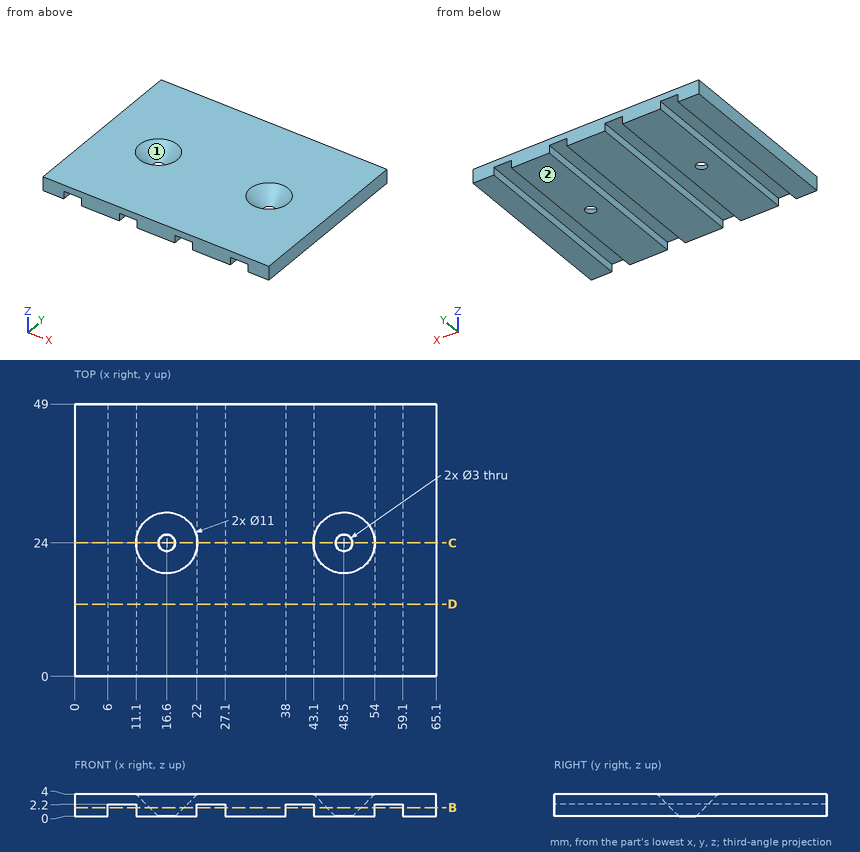
Study the drawing (mm; zero at the part's minimum x, y, z) and answer. Coordinates: 2 decimals unless noted, no trailing zeros. Write each loop counter-clockwise with the first axis right and the second up, starting at its lowest first coordinate (ties: lowest second). Pieces come first, ordered by that corner, then holes. Notation, with made-up numbers: (1.25, 76) - (56.25, 76) arc R25 cw to (56.25, 115) - close; hole circle Ø1 at (67.5, 9.25). An arc over 180 degrees is marked (long way). Answer as a JSON object with one key per item and string values. Group by question number.
1. The mould has two halves that part along X. Classify the marked faces 1 and 2: +X half, -X half, draft (parallel to the pull), parting line (faces both ways), or undercut.
2. Each of these flat-tipped pins is pushed along its axis until it touches: P1, Ø1.8, axis at y = 26, z = 1.5, coming from the -X side; P2, Ø2.5, axis at x = 24.5, y = 32, coming from the -Z side. Where does it stop, or does it pass through?
3. A cutting plane is placed at D-D (y = 13). Determine the outline of the cut face in (x, z), plus the area to 3 significant figures.
4. A cutting plane is placed at B-B (z = 1.6). Determine the outline of the cut face in (x, y).
5. Consider L1, parallel to X at y = 44.5, z = 0.2; L2, parallel to X at y = 23.5, z = 3.15; L3, parallel to Y at x = 13.5, z = 2.85. Determine where each line is inside the solid, lowest interval first. Write a range as [from, to].
6. A cutting plane is placed at C-C (y = 24). Give the number of separate pieces and of enclosed holes in the cut face, plus the area to 3 significant figures.
Worked out:
{
 "1": {"face 1": "undercut", "face 2": "draft"},
 "2": {"P1": "stops at x = 0", "P2": "stops at z = 2.2"},
 "3": {"outline": "(0, 0) - (6, 0) - (6, 2.2) - (11.1, 2.2) - (11.1, 0) - (22, 0) - (22, 2.2) - (27.1, 2.2) - (27.1, 0) - (38, 0) - (38, 2.2) - (43.1, 2.2) - (43.1, 0) - (54, 0) - (54, 2.2) - (59.1, 2.2) - (59.1, 0) - (65.1, 0) - (65.1, 4) - (0, 4) - close", "area": "216 mm²"},
 "4": {"outline": "(0, 0) - (6, 0) - (6, 49) - (0, 49) - close; (11.1, 0) - (22, 0) - (22, 49) - (11.1, 49) - close; (27.1, 0) - (38, 0) - (38, 49) - (27.1, 49) - close; (43.1, 0) - (54, 0) - (54, 49) - (43.1, 49) - close; (59.1, 0) - (65.1, 0) - (65.1, 49) - (59.1, 49) - close; hole circle Ø6.2 at (16.6, 24); hole circle Ø6.2 at (48.5, 24)"},
 "5": {"L1": "x = [0, 6], [11.1, 22], [27.1, 38], [43.1, 54], [59.1, 65.1]", "L2": "x = [0, 11.98], [21.22, 43.88], [53.12, 65.1]", "L3": "y = [0, 20.95], [27.05, 49]"},
 "6": {"separate pieces": "3", "enclosed holes": "0", "area": "160 mm²"}
}
